Could you check a few things on this model? Use its own coordinates, in mm. Face numbers are marked on the shaded views. A direction names the side the tool comes from. Give positions to 0.01 mm unless a question says otherwise; leave off trailing zeros. Order: outer loops, then holes, each group sorted by start corner. A loop starts at its lowest first (then second) coordinate and runs counter-clockwise, first axis right, second up.
(1) Imagine slicing it at D-D, the plane y = 10. Write out the boundary of the cut face in (x, z).
(2) Will these pins go through, and if not, where does the flat tip stop? pin 1 (6 mm diameter, centred on x = -1, y = 27, fed in from +Z); pin 2 (6.5 mm diameter, centred on x = 0, y = 26.5, fed in from +Z); pin 3 (2 mm diameter, centred on y = 11.5, z = 33, fed in from -X).
(3) On a 3-axis mill with a long thin cutter (end or side, diameter ignored), from which of +Z, -Z, +X, -X, +Y, -Y can I reach the whole of each face in a straight line? I mean the marked faces 1, 2 and 3. Say none if no direction works.
(4) Imagine slicing it at C-C, the plane z = 10. Write out the boundary of the cut face in (x, y).
(5) If I drill on probe 1 along Y at (x, z) = (0, 6.25); probe 2 along X at (y, z) = (12, 25); probe 3 along Y at (x, z) = (7, 13), over which ranges is the centre line in solid material (lowest first)?
(6) Imagine slicing it at B-B, the plane z = 30. Write out the boundary of the cut face in (x, y), then the cut area to 3 significant figures.
(7) If we mould it in two halves opening along Y, with no side actions, what happens to the marked faces 4, 5, 6 and 7? For each: released by +Y, released by -Y, zero draft, split by the parting line, or undercut.
(8) Imagine slicing it at A-A, the plane x = 0. Write out the boundary of the cut face in (y, z), then the cut area to 3 significant figures.
from build123d import *

# Parameters (mm, degrees)
EXTRUDE_1_DEPTH     = 15
CUT_EXTRUDE_1_DEPTH = 3.2
SKETCH_3_R          = 2.1
CUT_EXTRUDE_2_DEPTH = 38.739104388
SKETCH_1_4_W        = 4
SKETCH_1_4_H        = 20
EXTRUDE_2_DEPTH     = 40
SKETCH_4_R          = 2.1
CUT_EXTRUDE_6_DEPTH = 40
CHAMFER_1_SIZE      = 12
CUT_EXTRUDE_START   = -15
CUT_EXTRUDE_7_DEPTH = 3.2
CHAMFER_3_SIZE      = 0.5


with BuildPart() as part:
    # Sketch 1 → Extrude 1 (new body)
    with BuildSketch(Plane.XY):
        Polygon((-10, 33), (-10, 20), (10, 20), (14, 20), (14, 33), align=None)
    extrude(amount=EXTRUDE_1_DEPTH)

    # Sketch 2 → Cut-Extrude 1 (cut)
    with BuildSketch(Plane.XY.offset(15)):
        Polygon((4.156921938, 26.5), (2.078460969, 30.1), (-2.078460969, 30.1), (-4.156921938, 26.5), (-2.078460969, 22.9), (2.078460969, 22.9), align=None)
    extrude(amount=-CUT_EXTRUDE_1_DEPTH, mode=Mode.SUBTRACT)

    # Sketch 3 → Cut-Extrude 2 (cut, through all)
    with BuildSketch(Plane.XY.offset(11.8)):
        with Locations((0, 26.5)):
            Circle(SKETCH_3_R)
    extrude(amount=-CUT_EXTRUDE_2_DEPTH, mode=Mode.SUBTRACT)

    # Sketch 1_4 → Extrude 2 (add)
    with BuildSketch(Plane.XY):
        with Locations((12, 10)):
            Rectangle(SKETCH_1_4_W, SKETCH_1_4_H)
    extrude(amount=EXTRUDE_2_DEPTH)

    # Sketch 4 → Cut-Extrude 6 (cut)
    with BuildSketch(Plane(origin=(14, 0, 0), x_dir=(0, 0, -1), z_dir=(1, 0, 0))):
        with Locations((-30, 10)):
            Circle(SKETCH_4_R)
        with Locations((-10, 10)):
            Circle(SKETCH_4_R)
    extrude(amount=-CUT_EXTRUDE_6_DEPTH, mode=Mode.SUBTRACT)

    # Chamfer 1
    chamfer_1_edges = [part.edges().sort_by_distance(p)[0] for p in [
        (12, 20, 15),
    ]]
    chamfer(chamfer_1_edges, length=CHAMFER_1_SIZE)

    # Sketch 2_3 → Cut-Extrude 7 (cut)
    with BuildSketch(Plane.XY.offset(15).offset(CUT_EXTRUDE_START)):
        Polygon((4.156921938, 26.5), (2.078460969, 30.1), (-2.078460969, 30.1), (-4.156921938, 26.5), (-2.078460969, 22.9), (2.078460969, 22.9), align=None)
    extrude(amount=CUT_EXTRUDE_7_DEPTH, mode=Mode.SUBTRACT)

    # Chamfer 3
    chamfer_3_edges = [part.edges().sort_by_distance(p)[0] for p in [
        (2, 33, 15),
        (14, 20, 33.5),
        (14, 0, 20),
        (14, 10, 40),
        (14, 10, 32.1),
        (14, 10, 12.1),
        (2, 33, 0),
        (-10, 26.5, 15),
        (14, 32.5, 15),
        (14, 16.5, 0),
        (14, 26, 21),
        (-10, 26.5, 0),
        (-10, 33, 7.5),
        (14, 33, 7.5),
        (-10, 20, 7.5),
    ]]
    chamfer(chamfer_3_edges, length=CHAMFER_3_SIZE)


solid = part.part
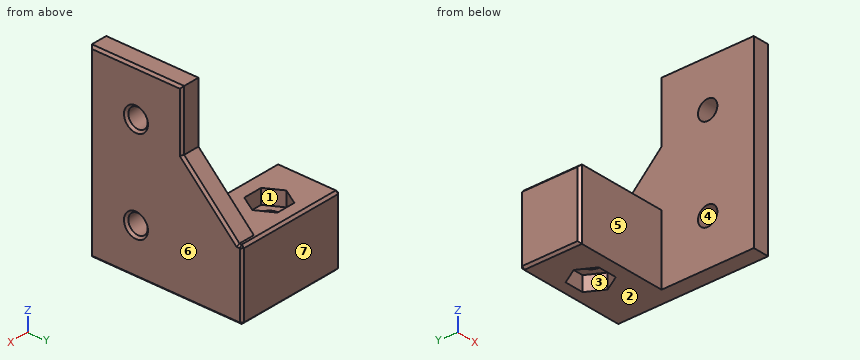
Answer block:
1. outline: (10, 0) - (13.5, 0) - (14, 0.5) - (14, 7.4) - (13.5, 7.9) - (10, 7.9) - close; (10, 12.1) - (13.5, 12.1) - (14, 12.6) - (14, 27.4) - (13.5, 27.9) - (10, 27.9) - close; (10, 32.1) - (13.5, 32.1) - (14, 32.6) - (14, 39.5) - (13.5, 40) - (10, 40) - close
2. pin 1: stops at z = 15
2. pin 2: stops at z = 11.8
2. pin 3: stops at x = 10
3. face 1: +Z
3. face 2: -Z, +X, -X, +Y, -Y
3. face 3: -Z
4. outline: (-10, 20.5) - (-9.5, 20) - (10, 20) - (10, 12.1) - (13.5, 12.1) - (14, 12.6) - (14, 32.5) - (13.5, 33) - (-9.5, 33) - (-10, 32.5) - close; (10, 0) - (13.5, 0) - (14, 0.5) - (14, 7.4) - (13.5, 7.9) - (10, 7.9) - close; hole circle Ø4.2 at (0, 26.5)
5. probe 1: y = 20 to 24.4, 28.6 to 33
5. probe 2: x = 10 to 14
5. probe 3: y = 20 to 33
6. outline: (10, 0) - (13.5, 0) - (14, 0.5) - (14, 7.4) - (13.5, 7.9) - (10, 7.9) - close; (10, 12.1) - (13.5, 12.1) - (14, 12.6) - (14, 19.5) - (13.5, 20) - (10, 20) - close
6. area: 62.7 mm2
7. face 4: undercut
7. face 5: released by -Y
7. face 6: zero draft
7. face 7: released by +Y
8. outline: (20, 0) - (22.9, 0) - (22.9, 3.2) - (24.4, 3.2) - (24.4, 11.8) - (22.9, 11.8) - (22.9, 15) - (20, 15) - close; (28.6, 3.2) - (30.1, 3.2) - (30.1, 0) - (32.5, 0) - (33, 0.5) - (33, 14.5) - (32.5, 15) - (30.1, 15) - (30.1, 11.8) - (28.6, 11.8) - close
8. area: 113 mm2
